Read the model definition and answer for the solid it produces. Units are mm, in the model's axes. A direction names the side the tool comes from. Give positions to 0.01 mm unless a question says otherwise; leave off trailing zeros. Order: outer loops, then holes, each group sorted by start corner. A loop starts at its lowest first (then second) coordinate and runs counter-clockwise, first axis right, second up. Notation, with made-up numbers: (-1, -34) -> (12, -34) arc R32 ccw to (12, 3) -> close; hole circle Ø2 at (27, 18.25). An arc over 180 degrees is marked (long way). One line per item, written item: value. Start each with the question number.
from build123d import *

# Parameters (mm, degrees)
F2_R     = 1.5875
F3_DEPTH = 25.4
F5_DEPTH = 3.175


with BuildPart() as f1:
    # F0 (on Right) → F1 (revolve)
    with BuildSketch(Plane.YZ):
        Polygon((0, 11.1125), (0, 6.94182), (32.9438, 6.7437), (32.9438, 6.3881), (36.8554, 6.1976), (339.725, 6.1976), (339.725, 11.1125), (327.025, 11.1125), (327.025, 13.17625), (193.675, 13.17625), (193.675, 15.24), (6.35, 15.24), (6.35, 11.1125), align=None)
    revolve(axis=Axis((0, 169.8625, 0), (0, -1, 0)))

    # F2 (on Top) → F3 (cut)
    with BuildSketch(Plane.XY):
        with Locations((0, 355.6)):
            Circle(F2_R)
    extrude(amount=F3_DEPTH, mode=Mode.SUBTRACT)

    # F4 (on face) → F5 (cut)
    with BuildSketch(Plane.XZ):
        Polygon((9.192321, 9.192321), (0, 0), (14.158506, -14.158506), (23.104484, -14.158506), (23.104484, 9.648457), align=None)
    extrude(amount=-F5_DEPTH, mode=Mode.SUBTRACT)


solid = f1.part
Item 1: Find the intervals of material crossed by line 1 (X direction, y = 126.5, z = 0); line 2 (Z direction, x = -0.5, y = 122.5); line 3 (Z direction, x = -4, y = 199), in increasing order. Write a range as from..to.
Item 2: For a pull along Z with two mould halves and no side action, classify faces 1 (the conical face through (5.563, 35.362, 2.893)), 2 (the cylindrical face through (-3.34, 333.29, 10.6)), 3 (the flat face through (9, 327.025, 7)) as +Z half, -Z half, draft (parallel to the pull), parting line (faces both ways), or undercut.
Item 3: A tool of negligible diameter and unlimited length cuts with its end or side. For faces 4 (the flat face through (5, 339.725, -5)), 5 (the flat face through (8, 3.175, 0)), 6 (the conical face through (-6.783, 16.703, -0.891)), 7 (the flat face through (-10, 193.675, 9)), from which of +Z, -Z, +X, -X, +Y, -Y can it reach the whole face along a straight path? Write none if from no direction.
Item 4: Flat-ended cylindrical pins translate along their axes: pin 1 (8 mm diameter, centred on x = 8, y = 194.5, fed in from +Z); pin 2 (1 mm diameter, centred on x = -8.5, y = 238, fed in from -Z); pin 3 (8 mm diameter, centred on x = 0, y = 236.5, fed in from +Z). Find the tip coordinate at first contact, or state that the pin passes through.
Item 5: Find section A-A on y = 172. Write down the section's boundary in (x, z), then the cut area to 3 significant figures.
Item 6: Find section B-B on y = 227. Write down the section's boundary in (x, z).
Checks:
1. line 1: -15.24..-6.2, 6.2..15.24
1. line 2: -15.23..-6.18, 6.18..15.23
1. line 3: -12.55..-4.73, 4.73..12.55
2. face 1: undercut
2. face 2: parting line
2. face 3: draft
3. face 4: +Z, -Z, +X, -X, +Y
3. face 5: +X, -Y
3. face 6: -Y
3. face 7: +Y
4. pin 1: z = 14.68
4. pin 2: z = -10.47
4. pin 3: z = 13.18
5. outline: circle Ø30.48 at (0, 0); hole circle Ø12.4 at (0, 0)
5. area: 609 mm2
6. outline: circle Ø26.35 at (0, 0); hole circle Ø12.4 at (0, 0)
